Could you check a few things on this drawing? It's one solid part, dimensions in mm from its lowest x, y, z. A direction names the side the tool comes from. Round coordinates to 2 decimals unless told otherwise and drop trailing zeros. Write each loop counter-clockwise with the first axis right and the second up, starting at its lowest first coordinate (ties: lowest second). Pieces come first, ordered by that corner, then holes. Notation, with made-up numbers: (6, -16) -> (34, -16) arc R10 ccw to (34, 2) -> close; hole circle Ø6 at (23.25, 17.5). An arc over 180 degrees is marked (long way). Return JSON: item names as keys, results as strings.
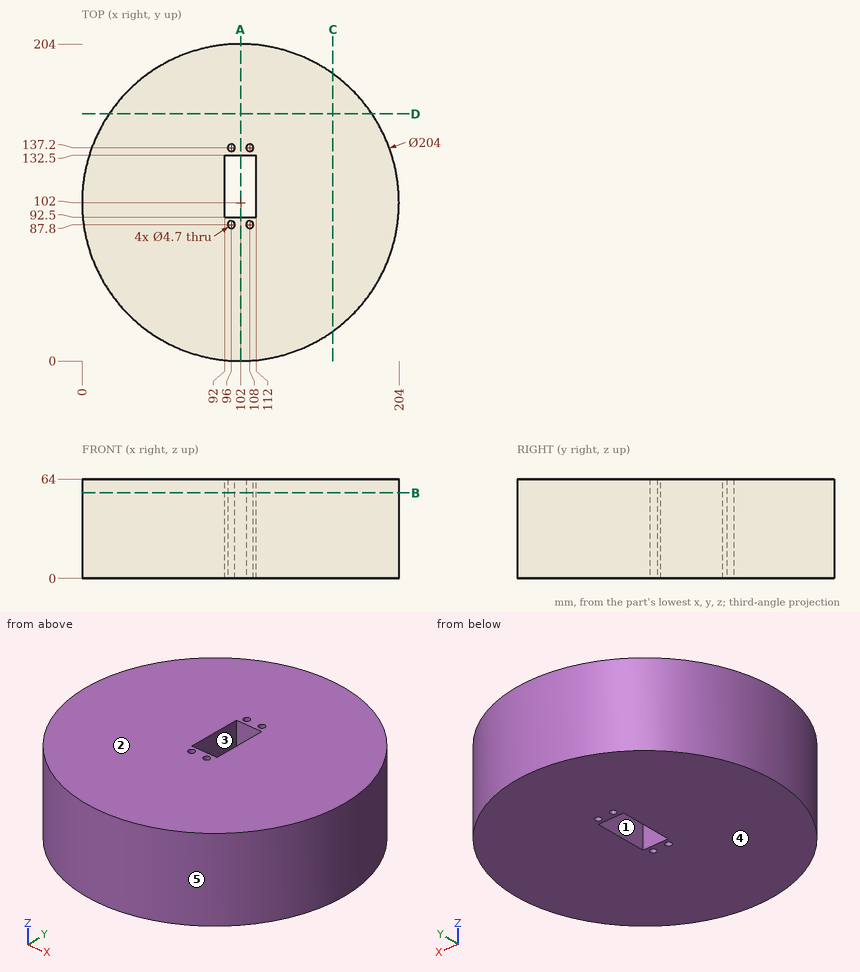
1) I want a section at B-B, the plane z = 55. Please give me the cut outline in (x, y).
Return value:
{"outline": "circle Ø204 at (102, 102); hole (92, 92.5) -> (112, 92.5) -> (112, 132.5) -> (92, 132.5) -> close; hole circle Ø4.7 at (96, 87.8); hole circle Ø4.7 at (96, 137.2); hole circle Ø4.7 at (108, 87.8); hole circle Ø4.7 at (108, 137.2)"}
2) If I drill on probe 1 along X at (y, z) = (87, 23); probe 2 along Y at (x, z) = (108, 38); probe 3 along X at (y, z) = (137, 35), over which ranges is the centre line in solid material (lowest first)? Write a range as [from, to].
Return value:
{"probe 1": "[1.11, 93.79], [98.21, 105.79], [110.21, 202.89]", "probe 2": "[0.18, 85.45], [90.15, 92.5], [132.5, 134.85], [139.55, 203.82]", "probe 3": "[6.19, 93.66], [98.34, 105.66], [110.34, 197.81]"}
3) I want a section at C-C, the plane x = 161.5. Please give me the cut outline in (y, z), and give its area (3 significant figures).
Return value:
{"outline": "(19.15, 0) -> (184.85, 0) -> (184.85, 64) -> (19.15, 64) -> close", "area": "10,600 mm²"}
4) Thinking about a two-plate mould opening in Y: for the marked faces 3, 4 and 5, which applies, pulls with the +Y half, pulls with the -Y half, needs draft (parallel to the pull), parting line crosses it, or undercut?
Return value:
{"face 3": "undercut", "face 4": "needs draft", "face 5": "parting line crosses it"}
5) I want a section at D-D, the plane y = 159. Please give me the cut outline in (x, z), and give its area (3 significant figures).
Return value:
{"outline": "(17.41, 0) -> (186.59, 0) -> (186.59, 64) -> (17.41, 64) -> close", "area": "10,800 mm²"}
6) I want a section at A-A, the plane x = 102. Please give me the cut outline in (y, z).
Return value:
{"outline": "(0, 0) -> (92.5, 0) -> (92.5, 64) -> (0, 64) -> close; (132.5, 0) -> (204, 0) -> (204, 64) -> (132.5, 64) -> close"}
7) For the marked faces 1 and 2, which set-ups out of +Z, -Z, +X, -X, +Y, -Y let a thin tool reach every point of the face, with its end or its side?
Return value:
{"face 1": "+Z, -Z", "face 2": "+Z, +X, -X, +Y, -Y"}
8) Will these pins go through, and if not, where does the flat tip stop? pin 1 Ø20 at (y, z) = (116, 37.5) entering from -X; pin 2 Ø3 at (x, y) = (96, 87.8) entering from -Z; pin 3 Ø1 at (x, z) = (26, 53.5) entering from +Y; pin 4 Ø12 at (y, z) = (175, 29.5) entering from -X.
Return value:
{"pin 1": "x = 0.08", "pin 2": "through", "pin 3": "y = 170.58", "pin 4": "x = 25.09"}
